```python
from build123d import *

# Parameters (mm, degrees)
F0_W      = 189
F0_H      = 85
F1_DEPTH  = 40
F2_R      = 10
F3_DEPTH  = 39
F4_W      = 102.8933165297
F4_H      = 85
F5_DEPTH  = 40.001
F6_SIZE   = 5
F8_DEPTH  = 25
F10_DEPTH = 86.1076834703


# Not quite as in the source:
# - a feature names something its author has since deleted; it is built from what else it names


with BuildPart() as f1:
    # F0 (on Top) → F1 (new body)
    with BuildSketch(Plane.XY):
        Rectangle(F0_W, F0_H)
    extrude(amount=F1_DEPTH)

    # F2 (on face) → F3 (cut)
    with BuildSketch(Plane.XY.offset(40)):
        with Locations((-82.6875, 31.875)):
            Circle(F2_R)
        with Locations((-61.6875, 31.875)):
            Circle(F2_R)
        with Locations((-40.6875, 31.875)):
            Circle(F2_R)
        with Locations((-19.6875, 31.875)):
            Circle(F2_R)
        with Locations((-19.6875, 10.875)):
            Circle(F2_R)
        with Locations((-40.6875, 10.875)):
            Circle(F2_R)
        with Locations((-61.6875, 10.875)):
            Circle(F2_R)
        with Locations((-82.6875, 10.875)):
            Circle(F2_R)
        with Locations((-82.6875, -10.125)):
            Circle(F2_R)
        with Locations((-61.6875, -10.125)):
            Circle(F2_R)
        with Locations((-40.6875, -10.125)):
            Circle(F2_R)
        with Locations((-19.6875, -10.125)):
            Circle(F2_R)
        with Locations((-19.6875, -31.125)):
            Circle(F2_R)
        with Locations((-40.6875, -31.125)):
            Circle(F2_R)
        with Locations((-61.6875, -31.125)):
            Circle(F2_R)
        with Locations((-82.6875, -31.125)):
            Circle(F2_R)
    extrude(amount=-F3_DEPTH, mode=Mode.SUBTRACT)

    # F4 (on face) → F5 (cut, through all)
    with BuildSketch(Plane.XY.offset(40)):
        with Locations((43.0533417352, 0)):
            Rectangle(F4_W, F4_H)
    extrude(amount=-F5_DEPTH, mode=Mode.SUBTRACT)

    # F6
    f6_edges = [f1.edges().sort_by_distance(p)[0] for p in [
        (-94.5, 42.5, 20),
        (-8.393317, 42.5, 20),
        (-8.393317, -42.5, 20),
        (-94.5, -42.5, 20),
    ]]
    chamfer(f6_edges, length=F6_SIZE)

    # F7 (on face) → F8 (cut)
    with BuildSketch(Plane(origin=(0, 0, 0), x_dir=(1, 0, 0), z_dir=(0, 0, -1))):
        Polygon((-9.3933165297, -37.0857864376), (-9.3933165297, 37.0857864376), (-13.8075300921, 41.5), (-89.0857864376, 41.5), (-93.5, 37.0857864376), (-93.5, -37.0857864376), (-89.0857864376, -41.5), (-13.8075300921, -41.5), align=None)
    extrude(amount=-F8_DEPTH, mode=Mode.SUBTRACT)

    # F9 (on face) → F10 (cut, through all)
    with BuildSketch(Plane.YZ.offset(-8.3933165297)):
        with BuildLine():
            Line((-37.5, 0), (37.5, 0))
            ThreePointArc((37.5, 0), (0, 15), (-37.5, 0))
        make_face()
    extrude(amount=-F10_DEPTH, mode=Mode.SUBTRACT)


solid = f1.part
```
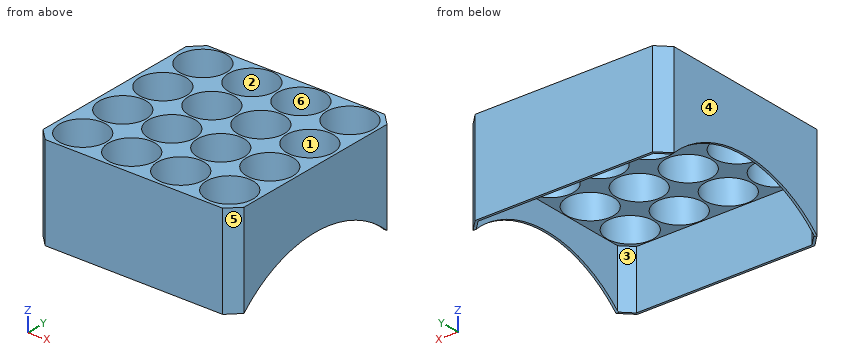
Geometry check sheet. Reference: the model listing, model coordinates, mm. Face numbers are marked on the shaded views. A direction names the side the tool comes from. Round coordinates to 2 decimals unless told otherwise and drop trailing zeros. Loops run counter-clockwise (first coordinate to the right, second up) from the corner with the lowest first, then second, coordinate; pieces in that order, holes last. Notation, with made-up numbers: (1.25, 20.25) - (32.25, 20.25) arc R14 ccw to (32.25, 47.25) - close; hole circle Ø6 at (-1, 16). An arc over 180 degrees is marked (long way). Write each question's results on one line, items separated by ' | '. Start each with the question number.
Q1. Cross-section at B-B on z = 35. State how many separate pieces and enclosed holes the cut face has, and give its area (3 significant figures).
Q2. Access from +Z, -Z, +X, -X, +Y, -Y to the whole of each face (thin tool, end or side, straight path). Record for the marked faces 1, 2 and 3.
Q3. Release check for a two-part mould opening along Y. For the marked faces 4, 5 and 6 record: +Y half, -Y half, draft (parallel to the pull), parting line (faces both ways), or undercut.
Q4. Cross-section at C-C on x = -74.5. Enter the section's corners in (y, z), and give its area (3 significant figures).
Q5. Cross-section at D-D on z = 17. Enter the section's corners in (x, y) (1 decimal).
Q6. Cross-section at A-A on y = 23.5. Enter the section's corners in (x, z).
Q7. Gauge pin test, flat ends, axial feed: P1, Ø12, axis at x = -61.69, y = -31.12, coming from the +Z side; P2, Ø10, axis at x = -77, y = 11.5, coming from the -Z side. Record the tip position at first contact, or that the pin passes through.
Q8. Thickness scan on line 1 (X direction, y = -10.5, z = 34.5); line 2 (Y direction, x = -19, z = 12); line 3 (Y direction, x = -41, z = 30.5). Record the ranges inside material, lowest first. Write a range as [from, to].
Answers below:
1) separate pieces: 1 | enclosed holes: 16 | area: 2,240 mm²
2) face 1: +Z, -Z | face 2: +Z | face 3: -Z
3) face 4: draft | face 5: -Y half | face 6: undercut
4) outline: (-42.5, 0) - (-41.5, 0) - (-41.5, 25) - (-36.87, 25) - (-36.87, 40) - (-42.5, 40) - close; (-25.38, 25) - (-15.87, 25) - (-15.87, 40) - (-25.38, 40) - close; (-4.38, 25) - (5.13, 25) - (5.13, 40) - (-4.38, 40) - close; (16.62, 25) - (26.13, 25) - (26.13, 40) - (16.62, 40) - close; (37.62, 25) - (41.5, 25) - (41.5, 0) - (42.5, 0) - (42.5, 40) - (37.62, 40) - close | area: 636 mm²
5) outline: (-94.5, -37.5) - (-89.5, -42.5) - (-13.4, -42.5) - (-8.4, -37.5) - (-8.4, 37.5) - (-13.4, 42.5) - (-89.5, 42.5) - (-94.5, 37.5) - close; hole (-93.5, -37.1) - (-89.1, -41.5) - (-13.8, -41.5) - (-9.4, -37.1) - (-9.4, 37.1) - (-13.8, 41.5) - (-17, 41.5) arc R10 ccw to (-22.4, 41.5) - (-38, 41.5) arc R10 ccw to (-43.4, 41.5) - (-59, 41.5) arc R10 ccw to (-64.4, 41.5) - (-80, 41.5) arc R10 ccw to (-85.4, 41.5) - (-89.1, 41.5) - (-93.5, 37.1) - close
6) outline: (-94.5, 9.66) - (-93.5, 9.66) - (-93.5, 25) - (-88.15, 25) - (-88.15, 40) - (-94.5, 40) - close; (-77.22, 25) - (-67.15, 25) - (-67.15, 40) - (-77.22, 40) - close; (-56.22, 25) - (-46.15, 25) - (-46.15, 40) - (-56.22, 40) - close; (-35.22, 25) - (-25.15, 25) - (-25.15, 40) - (-35.22, 40) - close; (-14.22, 25) - (-9.39, 25) - (-9.39, 9.66) - (-8.39, 9.66) - (-8.39, 40) - (-14.22, 40) - close
7) P1: passes through | P2: stops at z = 25
8) line 1: x = [-94.5, -92.68], [-72.69, -71.68], [-51.69, -50.68], [-30.69, -29.68], [-9.69, -8.39] | line 2: y = [-42.5, -41.5], [41.85, 42.5] | line 3: y = [-42.5, -41.12], [-21.13, -20.12], [-0.13, 0.88], [20.87, 21.88], [41.87, 42.5]
